from build123d import *

# Parameters (mm, degrees)
BOSS_EXTRUDE1_DEPTH     = 6.35
SKETCH2_R               = 2.6
CUT_EXTRUDE1_DEPTH      = 238.676928834
ESQUISSE3_R             = 21
ENL_V_MAT_EXTRU_2_DEPTH = 238.676928834
ESQUISSE7_R             = 1.5
ENL_V_MAT_EXTRU_3_DEPTH = 238.676928834
CUT_EXTRUDE3_DEPTH      = 238.676928834
SKETCH5_R               = 2
CUT_EXTRUDE4_DEPTH      = 238.676928834
SKETCH6_R               = 2
CUT_EXTRUDE5_DEPTH      = 238.676928834


with BuildPart() as part:
    # Sketch1 → Boss-Extrude1 (new body)
    with BuildSketch(Plane(origin=(0, 0, 0), x_dir=(1, 0, 0), z_dir=(0, 1, 0))):
        with BuildLine():
            Line((27.5, 0), (34.975254116, 198.684097441))
            ThreePointArc((34.975254116, 198.684097441), (0, 235), (-34.975254116, 198.684097441))
            Line((-34.975254116, 198.684097441), (-27.5, 0))
            ThreePointArc((-27.5, 0), (0, -27.5), (27.5, 0))
        make_face()
    extrude(amount=BOSS_EXTRUDE1_DEPTH)

    # Sketch2 → Cut-Extrude1 (cut, through all)
    with BuildSketch(Plane(origin=(0, 6.35, 0), x_dir=(1, 0, 0), z_dir=(0, 1, 0))):
        with Locations(Location((0, 0, 0), (0, 0, 270))):
            Circle(SKETCH2_R)
    extrude(amount=-CUT_EXTRUDE1_DEPTH, mode=Mode.SUBTRACT)

    # Esquisse3 → Enlèv. mat.-Extru.2 (cut, through all)
    with BuildSketch(Plane(origin=(0, 6.35, 0), x_dir=(1, 0, 0), z_dir=(0, 1, 0))):
        with Locations(Location((0, 200, 0), (0, 0, 270))):
            Circle(ESQUISSE3_R)
    extrude(amount=-ENL_V_MAT_EXTRU_2_DEPTH, mode=Mode.SUBTRACT)

    # Esquisse7 → Enlèv. mat.-Extru.3 (cut, through all)
    with BuildSketch(Plane(origin=(0, 6.35, 0), x_dir=(1, 0, 0), z_dir=(0, 1, 0))):
        with Locations(Location((-19.339370465, 219.339370465, 0), (0, 0, 270))):
            Circle(ESQUISSE7_R)
        with Locations(Location((19.339370465, 219.339370465, 0), (0, 0, 270))):
            Circle(ESQUISSE7_R)
        with Locations(Location((19.339370465, 180.660629535, 0), (0, 0, 270))):
            Circle(ESQUISSE7_R)
        with Locations(Location((-19.339370465, 180.660629535, 0), (0, 0, 270))):
            Circle(ESQUISSE7_R)
    extrude(amount=-ENL_V_MAT_EXTRU_3_DEPTH, mode=Mode.SUBTRACT)

    # Sketch4 → Cut-Extrude3 (cut, through all)
    with BuildSketch(Plane(origin=(0, 6.35, 0), x_dir=(1, 0, 0), z_dir=(0, 1, 0))):
        with BuildLine():
            Line((13.713919838, 60.073384505), (-16.927857887, 85.784888892))
            ThreePointArc((-16.927857887, 85.784888892), (-17.23599997, 89.306969024), (-13.713919838, 89.615111108))
            Line((-13.713919838, 89.615111108), (16.927857887, 63.90360672))
            ThreePointArc((16.927857887, 63.90360672), (17.23599997, 60.381526588), (13.713919838, 60.073384505))
        make_face()
    extrude(amount=-CUT_EXTRUDE3_DEPTH, mode=Mode.SUBTRACT)

    # Sketch5 → Cut-Extrude4 (cut, through all)
    with BuildSketch(Plane.XZ):
        with Locations(Location((-15.65, -113.2, 0), (0, 0, 90))):
            Circle(SKETCH5_R)
        with Locations(Location((15.35, -113.2, 0), (0, 0, 90))):
            Circle(SKETCH5_R)
        with Locations(Location((15.35, -144.2, 0), (0, 0, 90))):
            Circle(SKETCH5_R)
    extrude(amount=-CUT_EXTRUDE4_DEPTH, mode=Mode.SUBTRACT)

    # Sketch6 → Cut-Extrude5 (cut, through all)
    with BuildSketch(Plane(origin=(0, 6.35, 0), x_dir=(1, 0, 0), z_dir=(0, 1, 0))):
        with Locations(Location((-15.65, 144.2, 0), (0, 0, 270))):
            Circle(SKETCH6_R)
        with Locations(Location((-15.65, 113.2, 0), (0, 0, 270))):
            Circle(SKETCH6_R)
        with Locations(Location((15.35, 113.2, 0), (0, 0, 270))):
            Circle(SKETCH6_R)
        with Locations(Location((15.35, 144.2, 0), (0, 0, 270))):
            Circle(SKETCH6_R)
    extrude(amount=-CUT_EXTRUDE5_DEPTH, mode=Mode.SUBTRACT)


solid = part.part
Can you work these out from the model? Positions are in its coordinate system, mm. A direction names the side the tool comes from. Coordinates: 2 decimals unless noted, no trailing zeros. Order: outer loops, then holes, each group sorted by start corner. A loop starts at its lowest first (then second) coordinate and runs counter-clockwise, first axis right, second up. Notation, with made-up numbers: M 77,-32 L 115,-32 A14 cw 115,-26 Z; hole C 55.5,62 d1. An arc over 180 degrees is marked long. Answer as CSV lines item,"result".
(1) Suppose I cut it at A-A on x = 8.5. Please give me the cut outline in (y, z).
Geometry check:
outline,"M 0,-233.95 L 6.35,-233.95 L 6.35,-219.2 L 0,-219.2 Z; M 0,-180.8 L 6.35,-180.8 L 6.35,-70.98 L 0,-70.98 Z; M 0,-64.45 L 6.35,-64.45 L 6.35,26.15 L 0,26.15 Z"
(2) Suppose I cut it at B-B on z = -80.5. Please give me the cut outline in (x, y).
Geometry check:
outline,"M -30.53,0 L -10.63,0 L -10.63,6.35 L -30.53,6.35 Z; M -2.85,0 L 30.53,0 L 30.53,6.35 L -2.85,6.35 Z"
(3) Suppose I cut it at D-D on x = -10.5. Please give me the cut outline in (y, z).
Geometry check:
outline,"M 0,-233.39 L 6.35,-233.39 L 6.35,-218.19 L 0,-218.19 Z; M 0,-181.81 L 6.35,-181.81 L 6.35,-86.92 L 0,-86.92 Z; M 0,-80.39 L 6.35,-80.39 L 6.35,25.42 L 0,25.42 Z"
(4) On a 3-axis mill with a long thin cutter (end or side, diameter ignored), from which of +Z, -Z, +X, -X, +Y, -Y can I reach the whole of each face in a straight line? I mean faces 1 (the flat face through (0, 6.35, -106)), 2 (the flat face through (-1.392, 3.219, -72.749)). Say none if no direction works.
Geometry check:
face 1,"+Z, -Z, +X, -X, +Y"
face 2,"+Y, -Y"
(5) I'm going to push flat-ended pins straight in: pin 1 (1.5 mm diameter, centred on y = 2.5, z = -77.5, fed in from -X); pin 2 (2 mm diameter, centred on y = 5.5, z = -155.5, fed in from +X); pin 3 (1.5 mm diameter, centred on x = 6, y = 5, fed in from +Z). Where does each tip first touch, or does it pass through?
Geometry check:
pin 1,"x = -30.44"
pin 2,"x = 33.39"
pin 3,"z = 26.99"
(6) If we mould it in two halves opening along X, with no side actions, what happens to faces 3 (the flat face through (-31.29, 3.13, -100.73)), 4 (the flat face through (31.185, 3.131, -97.951)), 5 (the flat face through (0, 0, -106)), 6 (the cylindrical face through (0.78, 3.22, 2.48))? For each: released by +X, released by -X, zero draft, split by the parting line, or undercut.
Geometry check:
face 3,"released by -X"
face 4,"released by +X"
face 5,"zero draft"
face 6,"undercut"
(7) Suppose I cut it at C-C on y = 3. Count the separate pieces of the cut face and the enclosed holes in it, plus the area to 3 significant figures.
Geometry check:
separate pieces,"1"
enclosed holes,"11"
area,"13,900 mm^2"
(8) Please list where these lines run through material, in increasing order: L1, parallel to Z at x = 3, y = 0.5; L2, parallel to Z at x = 8, y = 2.75; L3, parallel to Z at x = 15.35, y = 4.5.
Geometry check:
L1,"-234.87 to -220.78, -179.22 to -75.59, -69.06 to 27.34"
L2,"-234.07 to -219.42, -180.58 to -71.39, -64.87 to 26.31"
L3,"-231.45 to -214.33, -185.67 to -146.2, -142.2 to -115.2, -111.2 to -65.23, -59.49 to 22.82"
